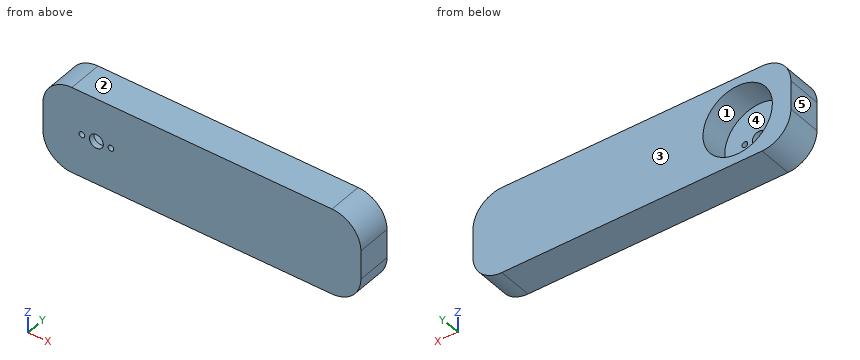
from build123d import *

# Parameters (mm, degrees)
SKETCH1_W           = 110
SKETCH1_H           = 30
BOSS_EXTRUDE1_DEPTH = 12
FILLET1_R           = 10
FILLET2_R           = 10
SKETCH9_R           = 12
CUT_EXTRUDE5_DEPTH  = 10
SKETCH10_R          = 2.4
SKETCH10_R_2        = 1
CUT_EXTRUDE6_DEPTH  = 64.95366743


with BuildPart() as part:
    # Sketch1 → Boss-Extrude1 (new body)
    with BuildSketch(Plane(origin=(0, 0, 0), x_dir=(1, 0, 0), z_dir=(0, 1, 0))):
        with Locations((5.385430756, 3.53837453)):
            Rectangle(SKETCH1_W, SKETCH1_H)
    extrude(amount=BOSS_EXTRUDE1_DEPTH)

    # Fillet1
    fillet1_edges = [part.edges().sort_by_distance(p)[0] for p in [
        (-49.614569244, 6, -18.53837453),
        (-49.614569244, 6, 11.46162547),
    ]]
    fillet(fillet1_edges, radius=FILLET1_R)

    # Fillet2
    fillet2_edges = [part.edges().sort_by_distance(p)[0] for p in [
        (60.385430756, 6, -18.53837453),
        (60.385430756, 6, 11.46162547),
    ]]
    fillet(fillet2_edges, radius=FILLET2_R)

    # Sketch9 → Cut-Extrude5 (cut)
    with BuildSketch(Plane(origin=(0, 12, 0), x_dir=(1, 0, 0), z_dir=(0, 1, 0))):
        with Locations(Location((-31.195762423, 3.53837453, 0), (0, 0, 270))):
            Circle(SKETCH9_R)
    extrude(amount=-CUT_EXTRUDE5_DEPTH, mode=Mode.SUBTRACT)

    # Sketch10 → Cut-Extrude6 (cut, through all)
    with BuildSketch(Plane(origin=(0, 2, 0), x_dir=(1, 0, 0), z_dir=(0, 1, 0))):
        with Locations(Location((-31.147671482, 3.53837453, 0), (0, 0, 270))):
            Circle(SKETCH10_R)
        with Locations(Location((-26.131792826, 3.53837453, 0), (0, 0, 270))):
            Circle(SKETCH10_R_2)
        with Locations(Location((-36.163550137, 3.53837453, 0), (0, 0, 90))):
            Circle(SKETCH10_R_2)
    extrude(amount=-CUT_EXTRUDE6_DEPTH, mode=Mode.SUBTRACT)


solid = part.part
Part model, mm, in its own coordinate system. Face numbers are marked on the shaded views. A direction names the side the tool comes from. Coordinates: 2 decimals unless noted, no trailing zeros. Order: outer loops, then holes, each group sorted by start corner. A loop starts at its lowest first (then second) coordinate and runs counter-clockwise, first axis right, second up.
(1) Slice it at C-C, the plane y = 10. Write the cut outline in (x, z), and give its area (3 significant figures).
Check sheet entries:
outline: (-49.61, -8.54) arc R10 ccw to (-39.61, -18.54) - (50.39, -18.54) arc R10 ccw to (60.39, -8.54) - (60.39, 1.46) arc R10 ccw to (50.39, 11.46) - (-39.61, 11.46) arc R10 ccw to (-49.61, 1.46) - close; hole circle Ø24 at (-31.2, -3.54)
area: 2,760 mm2
(2) Slice it at A-A, the plane z = -13.5. Write the cut outline in (x, y).
Check sheet entries:
outline: (-48.3, 0) - (59.07, 0) - (59.07, 12) - (-24.51, 12) - (-24.51, 2) - (-37.89, 2) - (-37.89, 12) - (-48.3, 12) - close
(3) Slice it at B-B, the plane y = 1. Write the cut outline in (x, z).
Check sheet entries:
outline: (-49.61, -8.54) arc R10 ccw to (-39.61, -18.54) - (50.39, -18.54) arc R10 ccw to (60.39, -8.54) - (60.39, 1.46) arc R10 ccw to (50.39, 11.46) - (-39.61, 11.46) arc R10 ccw to (-49.61, 1.46) - close; hole circle Ø2 at (-36.16, -3.54); hole circle Ø4.8 at (-31.15, -3.54); hole circle Ø2 at (-26.13, -3.54)
(4) Slice it at D-D, the plane z = 2.5. Write the cut outline in (x, y).
Check sheet entries:
outline: (-49.56, 0) - (60.33, 0) - (60.33, 12) - (-20.83, 12) - (-20.83, 2) - (-41.57, 2) - (-41.57, 12) - (-49.56, 12) - close
(5) Tool access for the marked faces 4 and 5: list every direction of +Z, -Z, +X, -X, +Y, -Y with a clear straight run to the whole face (end or side of a thin tool).
Check sheet entries:
face 4: +Y
face 5: +Z, -Z, -X, +Y, -Y
(6) Probe L1, parallel to X at y = 5.5, z = -6.75; L2, parallel to Z at x = -20.5, y = 10.25; L3, parallel to X at y = 11.25, z = -13.25. List the from-to ranges inside material, lowest first.
Check sheet entries:
L1: x = -49.61 to -42.76, -19.63 to 60.39
L2: z = -18.54 to -8.98, 1.9 to 11.46
L3: x = -48.44 to -38.24, -24.15 to 59.21
(7) Pull direction Z, two halves, no side cores. Call the marked faces 1, 2 and 3: pulls with the +Z half, pulls with the -Z half, needs draft (parallel to the pull), parting line crosses it, or undercut.
Check sheet entries:
face 1: undercut
face 2: pulls with the +Z half
face 3: needs draft
(8) Pin check, flat tips, straight feed: pin 1 Ø12 at (x, z) = (-26, -3) entering from +Y; pin 2 Ø4 at (y, z) = (1, 6.5) entering from -X. Stop position of each tip, or through.
Check sheet entries:
pin 1: stops at y = 2
pin 2: stops at x = -49.14
